Check sheet for the modelled part. Datum: model origin and axes. Units: mm. Round coordinates to 2 decimals unless told otherwise and drop trailing zeros. Loops run counter-clockwise (first coordinate to the right, second up) from the corner with the lowest first, then second, coordinate; pieces in that order, holes last. Notation, with made-up numbers: (33.5, -23) - (76.5, -23) arc R31 ccw to (76.5, 16) - close; hole circle Ø4 at (-1, -13.5). An arc over 180 degrees is marked (long way). Answer in a Markdown table with one row per item. Add a question column.
(1) Cross-section at D-D on x = 5. Count the separate pieces of the cut face and the enclosed holes in it, then the cut area to 3 significant figures.
(2) Cross-section at B-B on y = 6.25. Enter the section's corners in (x, z).
(3) Cross-section at C-C on y = 13.25. Enter the section's corners in (x, z).
(4) Gauge pin test, flat ends, axial feed: pin 1 (4 mm diameter, centred on x = -2.5, y = 12.5, fed in from +Z); pin 2 (1.5 mm diameter, centred on x = -7, y = 11, fed in from +Z); pin 3 (1.5 mm diameter, centred on x = 2, z = -1.5, fed in from -Y); pin 4 (5 mm diameter, centred on y = 16.5, z = -6, fed in from +X). Record the tip position at first contact, or that the pin passes through.
(5) Cross-section at A-A on x = 0. Enter the section's corners in (y, z).
(6) Mould release check, pull along X, two halves, no side actions. Record for faces 1 (the cylindrical face through (3.695, 12.328, 1.532)), 2 (the cylindrical face through (9.014, 12.328, -2.839)), 3 (the cylindrical face through (-6.62, 7.24, 0.13)): +X half, -X half, draft (parallel to the pull), parting line (faces both ways), or undercut.
(7) Thickness scan on line 1 along Y through (x, z) = (7, 0); line 2 along Z through (x, y) = (2.5, 19.75); line 3 along Z through (x, y) = (-5.85, 18.75). Record the ranges inside material, lowest first.
from build123d import *

# Parameters (mm, degrees)
SKETCH1_R           = 9.45
SKETCH1_R_2         = 4
BOSS_EXTRUDE1_DEPTH = 25
SKETCH2_R           = 1
CUT_EXTRUDE1_DEPTH  = 12.5
CHAMFER1_SIZE       = 0.25


with BuildPart() as part:
    # Sketch1 → Boss-Extrude1 (new body)
    with BuildSketch(Plane(origin=(0, 0, 0), x_dir=(1, 0, 0), z_dir=(0, 1, 0))):
        Circle(SKETCH1_R)
        Circle(SKETCH1_R_2, mode=Mode.SUBTRACT)
    extrude(amount=BOSS_EXTRUDE1_DEPTH)

    # Sketch2 → Cut-Extrude1 (cut, symmetric)
    with BuildSketch(Plane(origin=(0, 0, 0), x_dir=(0, 0, -1), z_dir=(1, 0, 0))):
        with Locations((0, 6.25)):
            Circle(SKETCH2_R)
        with Locations((0, 18.75)):
            Circle(SKETCH2_R)
    extrude(amount=CUT_EXTRUDE1_DEPTH, both=True, mode=Mode.SUBTRACT)

    # Chamfer1
    chamfer1_edges = [part.edges().sort_by_distance(p)[0] for p in [
        (-9.45, 0, 0),
        (-9.45, 25, 0),
        (-4, 0, 0),
        (-4, 25, 0),
    ]]
    chamfer(chamfer1_edges, length=CHAMFER1_SIZE)


solid = part.part
Answers:
| question | item | result |
|---|---|---|
| 1 | separate pieces | 1 |
| 1 | enclosed holes | 2 |
| 1 | area | 395 mm^2 |
| 2 | outline | (-9.4, -1) arc R9.45 ccw to (9.4, -1) - (3.87, -1) arc R4 cw to (-3.87, -1) - close; (-9.4, 1) - (-3.87, 1) arc R4 cw to (3.87, 1) - (9.4, 1) arc R9.45 ccw to start |
| 3 | outline | circle Ø18.9 at (0, 0); hole circle Ø8 at (0, 0) |
| 4 | pin 1 | stops at z = 9.44 |
| 4 | pin 2 | stops at z = 7.09 |
| 4 | pin 3 | passes through |
| 4 | pin 4 | stops at x = 8.78 |
| 5 | outline | (0, -9.2) - (0.25, -9.45) - (24.75, -9.45) - (25, -9.2) - (25, -4.25) - (24.75, -4) - (0.25, -4) - (0, -4.25) - close; (0, 4.25) - (0.25, 4) - (24.75, 4) - (25, 4.25) - (25, 9.2) - (24.75, 9.45) - (0.25, 9.45) - (0, 9.2) - close |
| 6 | face 1 | undercut |
| 6 | face 2 | parting line |
| 6 | face 3 | draft |
| 7 | line 1 | y = 0 to 5.25, 7.25 to 17.75, 19.75 to 25 |
| 7 | line 2 | z = -9.11 to -3.12, 3.12 to 9.11 |
| 7 | line 3 | z = -7.42 to -1, 1 to 7.42 |
